Drawing for the job (mm, zero at the part's lowest x, y, z). Coordinates: 2 decimals unless noted, no trailing zeros. Order: outer loops, then holes, each group sorted by start corner. A loop starts at its lowest first (then second) coordinate and runs counter-clockwise, first axis right, second up. Notation, with made-up numbers: M -17,-21.75 L 12,-21.75 A34 ccw 12,9.25 Z; hole C 12,40.25 d5. An arc over 180 degrees is marked long. Write item = value, one per line. Start each with the question number.
Q1. Band-saw the part on B-B on y = 6. Write the cut outline in (x, z).
Q2. Band-saw the part on C-C on z = 0.95. Write the cut outline in (x, y).
Q3. Drill centre lines: probe 1 along Y at (x, z) = (100, 3); probe 2 along Y at (x, z) = (57, 2.05); probe 3 along Y at (x, z) = (91.5, 2.7). Where is each one in solid material? Low to high.
Q4. Band-saw the part on D-D on x = 40.5. Write the cut outline in (y, z), plus the area to 3 significant figures.
Q5. Pin check, flat tip, straight feed: P1, Ø2, axis at x = 58, z = 1, coming from the +Y side. Stop position of the tip, or through.
Q6. Band-saw the part on A-A on x = 100. Write the cut outline in (y, z).
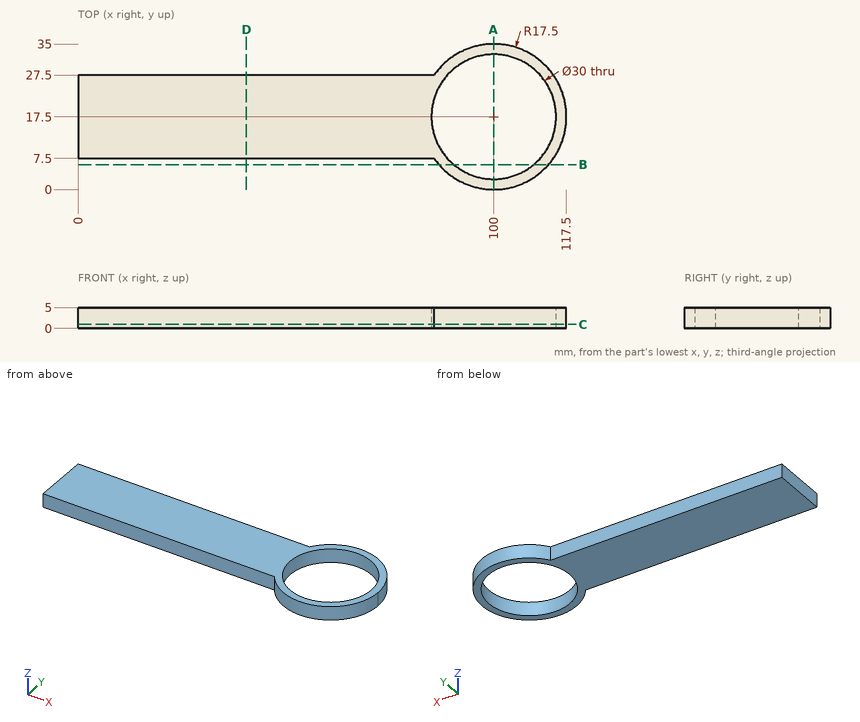
Recorded:
q1.outline = M 86.81,0 L 90.37,0 L 90.37,5 L 86.81,5 Z; M 109.63,0 L 113.19,0 L 113.19,5 L 109.63,5 Z
q2.outline = M 0,7.5 L 85.64,7.5 A17.5 ccw long 85.64,27.5 L 0,27.5 Z; hole C 100,17.5 d30
q3.probe_1 = 0 to 2.5, 32.5 to 35
q3.probe_2 = 7.5 to 27.5
q3.probe_3 = 2.2 to 5.14, 29.86 to 32.8
q4.outline = M 7.5,0 L 27.5,0 L 27.5,5 L 7.5,5 Z
q4.area = 100 mm2
q5.P1 = 27.5
q6.outline = M 0,0 L 2.5,0 L 2.5,5 L 0,5 Z; M 32.5,0 L 35,0 L 35,5 L 32.5,5 Z
